```python
from build123d import *

# Parameters (mm, degrees)
SKETCH_1_R          = 2.05
EXTRUDE_1_DEPTH     = 5
SKETCH_3_W          = 23.485848614
SKETCH_3_H          = 59.214320442
EXTRUDE_2_DEPTH     = 5
CUT_EXTRUDE_1_DEPTH = 4
FILLET_1_R          = 5


with BuildPart() as part:
    # 草圖1 → 填料-伸長1 (new, symmetric)
    with BuildSketch(Plane.XY):
        with BuildLine():
            Line((-30.167793166, 4.997183752), (14.832206834, 4.997183752))
            ThreePointArc((14.832206834, 4.997183752), (19.999295888, 0.083908399), (15, -5))
            Line((15, -5), (-30.167793166, -4.997183752))
            Line((-30.167793166, -4.997183752), (-55.167793166, -12.5))
            Line((-55.167793166, -12.5), (-55.167793166, 12.5))
            Line((-55.167793166, 12.5), (-30.167793166, 4.997183752))
        make_face()
        with Locations((15, 0)):
            Circle(SKETCH_1_R, mode=Mode.SUBTRACT)
    extrude(amount=EXTRUDE_1_DEPTH, both=True)

    # 草圖3 → 填料-伸長2 (add)
    with BuildSketch(Plane.ZY.offset(55.167793166)):
        Rectangle(SKETCH_3_W, SKETCH_3_H)
    extrude(amount=EXTRUDE_2_DEPTH)

    # 草圖4 → 除料-伸長1 (cut)
    with BuildSketch(Plane(origin=(0, 0, -5), x_dir=(-1, 0, 0), z_dir=(0, 0, -1))):
        Polygon((-16.638696654, -2.675834113), (-13.416200442, -2.938229795), (-11.57771101, -0.278664052), (-12.96171779, 2.643297373), (-16.184214003, 2.905693054), (-18.022703435, 0.246127311), align=None)
    extrude(amount=-CUT_EXTRUDE_1_DEPTH, mode=Mode.SUBTRACT)

    # 圓角1
    fillet_1_edges = [part.edges().sort_by_distance(p)[0] for p in [
        (-30.167793166, 4.997183752, 0),
        (-30.167793166, -4.997183752, 0),
        (-55.167793166, -12.5, 0),
        (-55.167793166, 12.5, 0),
        (-55.167793166, 0, -5),
        (-55.167793166, 0, 5),
    ]]
    fillet(fillet_1_edges, radius=FILLET_1_R)


solid = part.part
```
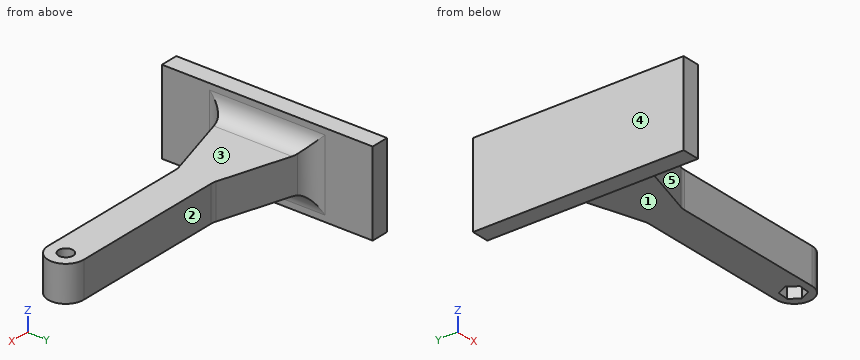
Input: part model. Units: mm. Frame: model coordinates. Face numbers are marked on the shaded views. A direction names the side the tool comes from. Coordinates: 2 decimals unless noted, no trailing zeros. Order: outer loops, then holes, each group sorted by start corner. A loop starts at its lowest first (then second) coordinate and runs counter-clockwise, first axis right, second up. Notation, with made-up numbers: (-36.75, 77.5) - (-22.75, 77.5) arc R29 cw to (-22.75, 102.5) - close; hole circle Ø5 at (22, 54). An arc over 180 degrees is marked (long way). Return JSON: item names as keys, results as strings.
Q1. Cut plane D-D (y = 8.5). Return loops of the section in (x, z).
The answers:
{"outline": "(-60.17, -11.74) - (-55.17, -11.74) - (-55.17, -10) arc R5 cw to (-50.17, -5) - (-41.84, -5) - (-41.84, 5) - (-50.17, 5) arc R5 cw to (-55.17, 10) - (-55.17, 11.74) - (-60.17, 11.74) - close"}
Q2. Access query for the marked faces 1, 2, 3, 4 and 5. Directions: +Z, -Z, +X, -X, +Y, -Y. A direction counts if a zero-diameter tool reaches every point of the face in a straight line with its end or side. Return the directions, or none.
The answers:
{"face 1": "-Z, +X, +Y, -Y", "face 2": "+Z, -Z, +X, +Y", "face 3": "+Z, +X, +Y, -Y", "face 4": "+Z, -Z, -X, +Y, -Y", "face 5": "+Z, -Z, +X, -Y"}
Q3. Cut plane B-B (y = -15). Return loops of the section in (x, z), then the cut area to 3 significant figures.
The answers:
{"outline": "(-60.17, -11.74) - (-55.17, -11.74) - (-55.17, -10) arc R5 cw to (-55.02, -8.78) - (-55.02, 8.78) arc R5 cw to (-55.17, 10) - (-55.17, 11.74) - (-60.17, 11.74) - close", "area": "120 mm2"}
Q4. Ray query, probe 1 along X at (y, z) = (0, 1.15); probe 2 along Y at (x, z) = (15, 3.2); probe 3 along Y at (x, z) = (2, 0.25). Return the intervals inside material, ascending.
The answers:
{"probe 1": "x = -60.17 to 12.95, 17.05 to 20", "probe 2": "y = -5 to -2.05, 2.05 to 5", "probe 3": "y = -5 to 5"}
Q5. Cut plane A-A (z = -2). Return loops of the section in (x, y), then the cut area to 3 significant figures.
The answers:
{"outline": "(-60.17, -29.61) - (-55.17, -29.61) - (-55.17, -16.22) arc R5 cw to (-51.61, -11.43) - (-30.87, -5.21) arc R5 cw to (-29.43, -5) - (15, -5) arc R5 ccw (long way) to (14.83, 5) - (-29.43, 5) arc R5 cw to (-30.87, 5.21) - (-51.61, 11.43) arc R5 cw to (-55.17, 16.22) - (-55.17, 29.61) - (-60.17, 29.61) - close; hole (11.58, -0.28) - (13.42, -2.94) - (16.64, -2.68) - (18.02, 0.25) - (16.18, 2.91) - (12.96, 2.64) - close", "area": "1,200 mm2"}
Q6. First-contact query: pin 1 (3 mm diameter, centred on y = -15, z = -5.5, fed in from +X); pin 2 (6.5 mm diameter, centred on x = 15, y = 1.5, fed in from -Z); pin 3 (5 mm diameter, centred on x = 1, z = -2, fed in from -Y). Flat tips, straight axial feed; report the tip coordinate or a pass-through.
The answers:
{"pin 1": "stops at x = -54.36", "pin 2": "stops at z = -5", "pin 3": "stops at y = -5"}
Q7. Cut plane C-C (x = -3.5). Return loops of the section in (y, z).
The answers:
{"outline": "(-5, -5) - (5, -5) - (5, 5) - (-5, 5) - close"}
